from build123d import *

# Parameters (mm, degrees)
F1_DEPTH = 130.175
F2_T     = -2.54
F0_R     = 3.81
F3_DEPTH = 1.27


with BuildPart() as f1:
    # F0 (on Front) → F1 (new body)
    with BuildSketch(Plane.XZ):
        with BuildLine():
            ThreePointArc((-179.94042, 32.1801), (-175.54974, -3.808035), (-168.499008, -39.370812))
            ThreePointArc((-168.499008, -39.370812), (41.747481, -167.321401), (167.244505, 44.398783))
            ThreePointArc((167.244505, 44.398783), (156.678782, 126.446336), (167.244505, 208.493888))
            Line((167.244505, 208.493888), (-181.670055, 74.106991))
            ThreePointArc((-181.670055, 74.106991), (-181.301912, 54.266409), (-180.127338, 34.457204))
            ThreePointArc((-180.127338, 34.457204), (-179.917292, 33.752862), (-179.846398, 33.021294))
            ThreePointArc((-179.846398, 33.021294), (-179.869976, 32.598078), (-179.94042, 32.1801))
        make_face()
    extrude(amount=F1_DEPTH)

    # F2
    f2_openings = [f1.faces().sort_by_distance(p)[0] for p in [
        (-7.212775, -65.0875, 141.30044),
    ]]
    offset(amount=F2_T, openings=f2_openings)

    # F0 (on Front) → F3 (join)
    with BuildSketch(Plane.XZ):
        with BuildLine():
            ThreePointArc((-191.19504, 74.123976), (-187.878519, 15.883128), (-177.76688, -41.56903))
            ThreePointArc((-177.76688, -41.56903), (44.053325, -176.563085), (176.458749, 46.81194))
            ThreePointArc((176.458749, 46.81194), (166.203782, 126.446336), (176.458749, 206.080731))
            ThreePointArc((176.458749, 206.080731), (177.970177, 211.454842), (179.674253, 216.771007))
            Line((179.674253, 216.771007), (-191.19504, 74.123976))
        make_face()
        with Locations((-124.498114, -126.301363)):
            Circle(F0_R, mode=Mode.SUBTRACT)
        with Locations((-63.980319, -164.931968)):
            Circle(F0_R, mode=Mode.SUBTRACT)
        with Locations((-166.418388, -62.232696)):
            Circle(F0_R, mode=Mode.SUBTRACT)
        with Locations((14.358005, -176.30595)):
            Circle(F0_R, mode=Mode.SUBTRACT)
        with Locations((80.824465, -157.232255)):
            Circle(F0_R, mode=Mode.SUBTRACT)
        with Locations((135.350421, -113.461576)):
            Circle(F0_R, mode=Mode.SUBTRACT)
        with Locations((172.669113, -39.752249)):
            Circle(F0_R, mode=Mode.SUBTRACT)
        with BuildLine():
            ThreePointArc((167.244505, 44.398783), (41.747481, -167.321401), (-168.499008, -39.370812))
            ThreePointArc((-168.499008, -39.370812), (-175.54974, -3.808035), (-179.94042, 32.1801))
            ThreePointArc((-179.94042, 32.1801), (-187.453626, 32.709595), (-180.127338, 34.457204))
            ThreePointArc((-180.127338, 34.457204), (-181.301912, 54.266409), (-181.670055, 74.106991))
            Line((-181.670055, 74.106991), (167.244505, 208.493888))
            ThreePointArc((167.244505, 208.493888), (156.678782, 126.446336), (167.244505, 44.398783))
        make_face(mode=Mode.SUBTRACT)
        with Locations((163.721606, 91.117166)):
            Circle(F0_R, mode=Mode.SUBTRACT)
    extrude(amount=F3_DEPTH)

    # F5: F1 across plane


with BuildPart() as f1_1:
    add(f1.part)
    add(f1.part.mirror(Plane.XZ.offset(65.0875)))


solid = f1_1.part
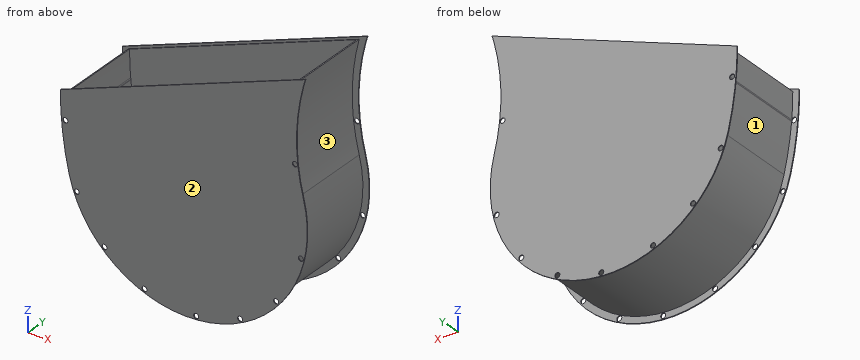
CAD build for the part. Positions are in the model's coordinates, mm. Face numbers are marked on the shaded views. Round coordinates to 2 decimals unless told otherwise and drop trailing zeros. Order: outer loops, then holes, each group sorted by start corner. A loop starts at its lowest first (then second) coordinate and runs counter-clockwise, first axis right, second up. Notation, with made-up numbers: (9, 67) -> (52, 67) arc R23 cw to (52, 106) -> close; hole circle Ø8 at (26, 3.25). An arc over 180 degrees is marked (long way). Write each question's results on one line, items separated by ' | '.
1. Flat gauge pins, fed straight in: P1, Ø5, axis at y = -103.5, z = -134, coming from the +X side; P2, Ø12, axis at x = -124.5, z = -126.3, coming from the -Y side (3 decimals); P3, Ø12, axis at x = -83, y = -45, coming from the -Z side; P4, Ø6, axis at y = -17.5, z = 19, coming from the +X side. Where does each tip first touch, or does it go through?
Findings below:
P1: stops at x = 111.66 | P2: stops at y = -130.175 | P3: stops at z = -154.46 | P4: stops at x = 172.2
2. Wall check: line 1 along Y through (x, z) = (123.5, 129) (3 decimals); line 2 along Y through (x, z) = (-145, -105) (3 decimals); line 3 along X through (y, z) = (-10.5, 30.5). Give the ranges that are in metal, low to high. Write a range as [from, to].
Findings below:
line 1: y = [-130.175, -127.635], [-2.54, 0] | line 2: y = [-130.175, -128.905], [-1.27, 0] | line 3: x = [-179.8, -177.25], [167.7, 170.28]
3. Cut at A-A (z = 23). Give the cut face in (x, y) (3 decimals), plus the area to 3 significant figures.
Findings below:
outline: (-188.653, -130.175) -> (181.03, -130.175) -> (181.03, -128.905) -> (171.429, -128.905) -> (171.429, -1.27) -> (181.03, -1.27) -> (181.03, 0) -> (-188.653, 0) -> (-188.653, -1.27) -> (-179.078, -1.27) -> (-179.078, -128.905) -> (-188.653, -128.905) -> close; hole (-176.524, -127.635) -> (168.867, -127.635) -> (168.867, -2.54) -> (-176.524, -2.54) -> close | area: 2,470 mm²
4. Pull direction Z, two halves, no side cores. Call the marked faces 1, 2 and 3: pulls with the +Z half, pulls with the -Z half, needs draft (parallel to the pull), parting line crosses it, or undercut.
Findings below:
face 1: pulls with the -Z half | face 2: needs draft | face 3: undercut
5. Cut at D-D (z = 128). Give the cut face in (x, y) (1 decimal).
Findings below:
outline: (-51.1, -130.2) -> (166.2, -130.2) -> (166.2, -128.9) -> (156.7, -128.9) -> (156.7, -1.3) -> (166.2, -1.3) -> (166.2, 0) -> (-51.1, 0) -> (-51.1, -1.3) -> (-41.7, -1.3) -> (-41.7, -2.5) -> (154.1, -2.5) -> (154.1, -127.6) -> (-41.7, -127.6) -> (-41.7, -128.9) -> (-51.1, -128.9) -> close
6. Cut at C-C (x = 114). Give the cut face in (y, z) (3 decimals).
Findings below:
outline: (-130.175, -141.91) -> (-128.905, -141.91) -> (-128.905, -129.482) -> (-1.27, -129.482) -> (-1.27, -141.91) -> (0, -141.91) -> (0, 191.511) -> (-1.27, 191.511) -> (-1.27, 187.986) -> (-2.54, 187.986) -> (-2.54, -126.083) -> (-127.635, -126.083) -> (-127.635, 187.986) -> (-128.905, 187.986) -> (-128.905, 191.511) -> (-130.175, 191.511) -> close
